Input: part model. Units: mm. Frame: model coordinates. Coordinates: 2 decimals unless noted, no trailing zeros. Write each loop counter-clockwise with the first axis right and the second up, starting at its lowest first coordinate (ties: lowest second). Pieces come first, ordered by that corner, then holes. Notation, with made-up numbers: M -29,-31.5 L 12,-31.5 A21 ccw 12,-4.5 Z; hole C 58,64.25 d6. An arc over 180 degrees is marked long. Use CSV: the item, a comma, the result in double quotes.
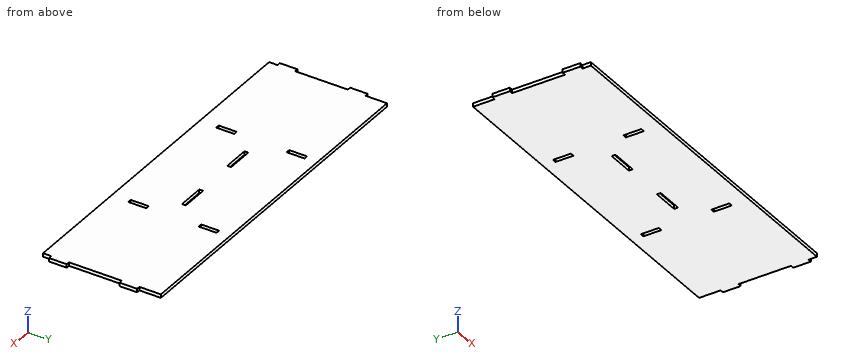
```python
from build123d import *

# Parameters (mm, degrees)
SKETCH_1_W      = 4.4
SKETCH_1_H      = 20.4
SKETCH_1_W_2    = 30.4
SKETCH_1_H_2    = 4.4
EXTRUDE_1_DEPTH = 4


with BuildPart() as part:
    # Эскиз1 → Бобышка-Вытянуть1 (new body)
    with BuildSketch(Plane.XY):
        Polygon((0, 9.5), (0, 0), (400, 0), (400, 9.5), (404, 9.5), (404, 29.5), (400, 29.5), (400, 89.5), (404, 89.5), (404, 109.5), (400, 109.5), (400, 134), (0, 134), (0, 109.5), (-4, 109.5), (-4, 89.5), (0, 89.5), (0, 29.5), (-4, 29.5), (-4, 9.5), align=None)
        with Locations((122.2, 30)):
            Rectangle(SKETCH_1_W, SKETCH_1_H, mode=Mode.SUBTRACT)
        with Locations((277.8, 30)):
            Rectangle(SKETCH_1_W, SKETCH_1_H, mode=Mode.SUBTRACT)
        with Locations((160, 67.2)):
            Rectangle(SKETCH_1_W_2, SKETCH_1_H_2, mode=Mode.SUBTRACT)
        with Locations((122.2, 110)):
            Rectangle(SKETCH_1_W, SKETCH_1_H, mode=Mode.SUBTRACT)
        with Locations((240, 67.2)):
            Rectangle(SKETCH_1_W_2, SKETCH_1_H_2, mode=Mode.SUBTRACT)
        with Locations((277.8, 110)):
            Rectangle(SKETCH_1_W, SKETCH_1_H, mode=Mode.SUBTRACT)
    extrude(amount=EXTRUDE_1_DEPTH)


solid = part.part
```
1. Section B-B (z = 1.8). State how many separate pieces and enclosed holes the cut face has, then the cut area to 3 significant figures.
Resolved:
separate pieces,"1"
enclosed holes,"6"
area,"53,300 mm^2"
2. Material intervals for line 1 (X direction, y = 108, z = 3.65); line 2 (X direction, y = 37.5, z = 0.5); line 3 (Y direction, x = 225, z = 3.2), sorted ascending. Write a range as [from, to].
Resolved:
line 1,"x = [-4, 120], [124.4, 275.6], [280, 404]"
line 2,"x = [0, 120], [124.4, 275.6], [280, 400]"
line 3,"y = [0, 65], [69.4, 134]"
3. Section C-C (y = 55). Return loops of the section in (x, z), then the cut area to 3 significant figures.
Resolved:
outline,"M 0,0 L 400,0 L 400,4 L 0,4 Z"
area,"1,600 mm^2"
4. Contact query for flat-ended pins moving along their axis: pin 1 Ø1.2 at (y, z) = (34, 2.5) entering from +X; pin 2 Ø2 at (x, z) = (402, 2) entering from -Y. Output: stop coordinate, or through.
Resolved:
pin 1,"stops at x = 400"
pin 2,"stops at y = 9.5"
5. Section A-A (x = 235.5). Return loops of the section in (y, z), then the cut area to 3 significant figures.
Resolved:
outline,"M 0,0 L 65,0 L 65,4 L 0,4 Z; M 69.4,0 L 134,0 L 134,4 L 69.4,4 Z"
area,"518 mm^2"
